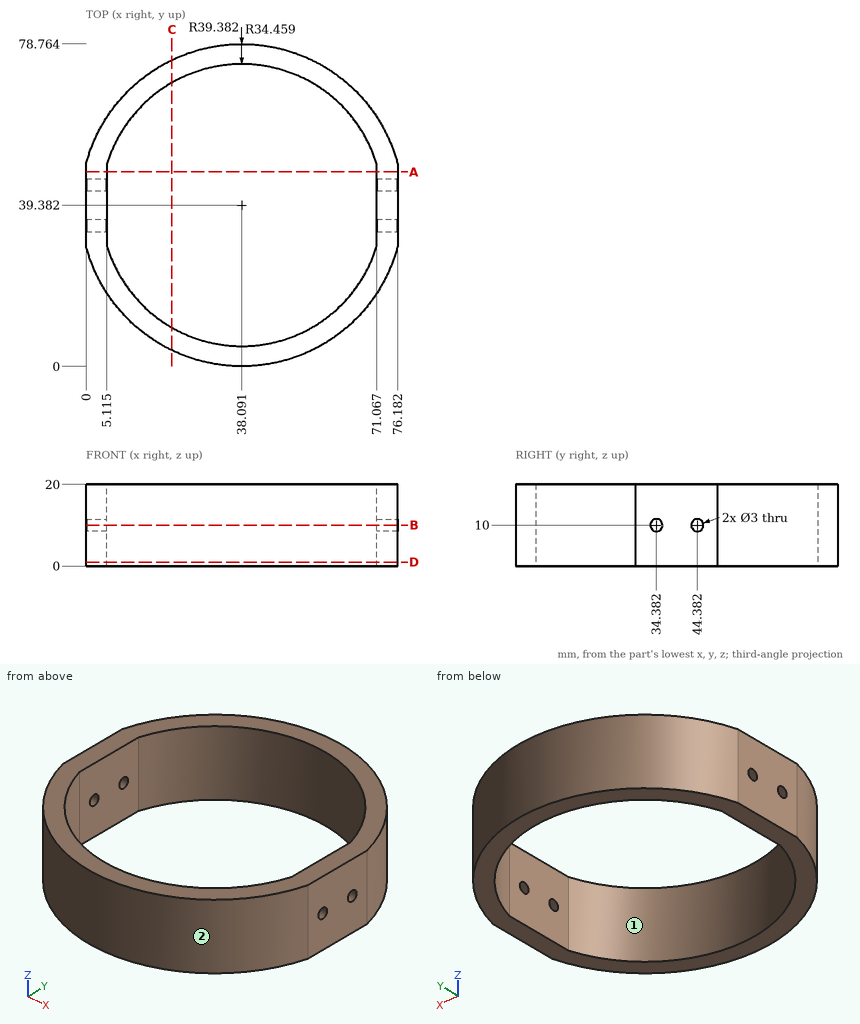
The figure shows three views and two pictorial views of one solid part (mm, origin at its lowest corner). Answer the questions. A direction names the side the tool comes from. Give positions to 0.01 mm unless a question says otherwise; leave off trailing zeros. Loops run counter-clockwise (first coordinate to the right, second up) from the corner with the lowest first, then second, coordinate; pieces in that order, holes last. Notation, with made-up numbers: (61, -23) -> (109, -23) arc R13 cw to (109, -2) -> close; hole circle Ø7 at (-35, 30.25). An arc over 180 degrees is marked (long way). Put each result on its own line as item: value. Start each with the question number.
Item 1: The part is cut by section C-C (x = 21). Give the vertices of the cut face in (y, z).
Item 2: The part is cut by section D-D (z = 1). Give the vertices of the cut face in (x, y) (1 decimal), then the cut area to 3 significant figures.
Item 3: Each of these flat-tipped pins is pushed along its axis until it touches: P1, Ø2, axis at x = 20, z = 2.5, coming from the -Y side; P2, Ø5, axis at y = 19, z = 6.5, coming from the -X side; P3, Ø1, axis at y = 13, z = 3, coming from the +X side (1 decimal). Where does it stop, or does it pass through?
Item 4: The part is cut by section A-A (y = 47.5). Give the vertices of the cut face in (x, z) (1 decimal).
Item 5: The part is cut by section B-B (z = 10). Give the vertices of the cut face in (x, y) (1 decimal).
Item 6: Which of the six approach directions +Z, -Z, +X, -X, +Y, -Y give full straight-line access (tool end or side, diameter ignored) to the marked faces 1 and 2?
Item 7: Find the intervals of material crossed by L1, parallel to X at y = 46.5, z = 11.75 (1 decimal); L2, parallel to Y at x = 2.7, z = 10 (1 decimal); L3, parallel to Y at x = 2.75, z = 10 (1 decimal), in increasing order. Write a range as [from, to].
Answers below:
1. outline: (3.9, 0) -> (9.46, 0) -> (9.46, 20) -> (3.9, 20) -> close; (69.3, 0) -> (74.86, 0) -> (74.86, 20) -> (69.3, 20) -> close
2. outline: (0, 29.4) arc R39.4 ccw to (76.2, 29.4) -> (76.2, 49.4) arc R39.4 ccw to (0, 49.4) -> close; hole (5.1, 29.4) arc R34.5 ccw to (71.1, 29.4) -> (71.1, 49.4) arc R34.5 ccw to (5.1, 49.4) -> close
2. area: 1,150 mm2
3. P1: y = 3.9
3. P2: x = 3
3. P3: x = 67.8
4. outline: (0, 0) -> (5.1, 0) -> (5.1, 20) -> (0, 20) -> close; (71.1, 0) -> (76.2, 0) -> (76.2, 20) -> (71.1, 20) -> close
5. outline: (0, 29.4) arc R39.4 ccw to (76.2, 29.4) -> (76.2, 32.9) -> (71.1, 32.9) -> (71.1, 29.4) arc R34.5 cw to (5.1, 29.4) -> (5.1, 32.9) -> (0, 32.9) -> close; (0, 35.9) -> (5.1, 35.9) -> (5.1, 42.9) -> (0, 42.9) -> close; (0, 45.9) -> (5.1, 45.9) -> (5.1, 49.4) arc R34.5 cw to (71.1, 49.4) -> (71.1, 45.9) -> (76.2, 45.9) -> (76.2, 49.4) arc R39.4 ccw to (0, 49.4) -> close; (71.1, 35.9) -> (76.2, 35.9) -> (76.2, 42.9) -> (71.1, 42.9) -> close
6. face 1: +Z, -Z
6. face 2: +Z, -Z, -Y
7. L1: [0, 5.1], [71.1, 76.2]
7. L2: [22.1, 32.9], [35.9, 42.9], [45.9, 56.7]
7. L3: [22, 32.9], [35.9, 42.9], [45.9, 56.8]
